Geometry: final body of the model. Coordinates: model frame, mm. Face numbers are marked on the shaded views. A direction names the side the tool comes from. Give positions to 0.01 mm unless a question says otherwise; leave off trailing zeros. Loops run counter-clockwise (first coordinate to the right, second up) from the corner with the lowest first, then second, coordinate; pieces in that order, holes last. Notation, with made-up numbers: (-13, -4) -> (7, -4) arc R14 cw to (7, 23) -> close; hole circle Ø6 at (-21.5, -34). An arc over 180 degrees is marked (long way). One line per question, with ' | ' between items. Start each with the question number.
Item 1: Pin query (flat end, axial travel): P1, Ø10, axis at x = -14, z = 4.5, coming from the +Y side; P2, Ø23, axis at y = 32, z = 0, coming from the -X side; P3, Ø8, axis at x = -27, z = 9, coming from the -Y side. Return the tip coordinate at first contact, or that it passes through.
Item 2: Set-up query: the marked faces 1, 2 and 3. Return all of +Z, -Z, +X, -X, +Y, -Y with unobstructed straight access to the full face (end or side cutting, diameter ignored); none if empty.
Item 3: Section B-B on z = 2. Return loops of the section in (x, y), then the cut area to 3 significant figures.
Item 4: Mould query, pull axis X, two halves, no side actions, for the marked faces 4, 5, 6 and 7. Classes: released by +X, released by -X, zero draft, split by the parting line, or undercut.
Item 5: Material intervals for line 1 along X through (y, z) = (5, -1); line 2 along X through (y, z) = (-1.5, -2); line 3 along Z through (x, y) = (-25, 2.75), sorted ascending. Write a range as [from, to].
Item 6: Section C-C on y = 36. Return loops of the section in (x, z), then the cut area to 3 significant figures.
Item 7: Section A-A on x = -25. Return loops of the section in (y, z).
Item 8: Section D-D on x = -43. Return loops of the section in (y, z).
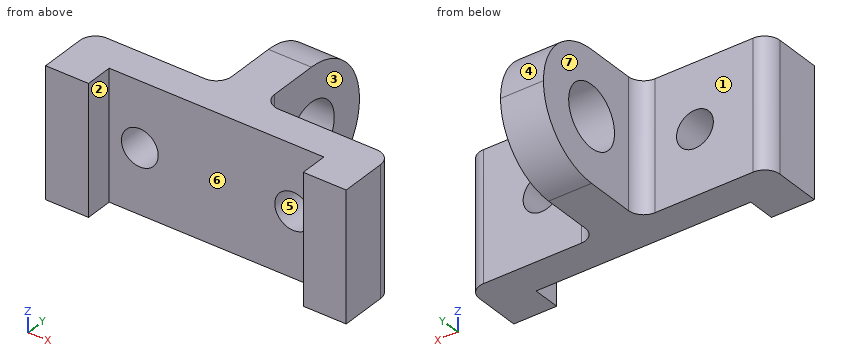
from build123d import *

# Parameters (mm, degrees)
SKETCH2_W               = 98
SKETCH2_H               = 42
BOSS_EXTRUDE1_DEPTH     = 11
SKETCH3_W               = 14
SKETCH3_H               = 42
BOSS_EXTRUDE2_DEPTH     = 9
FILLET1_R               = 5
CUT_EXTRUDE1_DEPTH      = 55.433445601
CUT_EXTRUDE1_DEPTH_BACK = 55.433445601
SKETCH4_R               = 6
SKETCH5_W               = 14
SKETCH5_H               = 42
BOSS_EXTRUDE4_DEPTH     = 53
FILLET2_R               = 21
FILLET3_R               = 5
CUT_EXTRUDE2_DEPTH      = 76.173133499
CUT_EXTRUDE2_DEPTH_BACK = 76.173133499
SKETCH6_R               = 10


with BuildPart() as part:
    # Sketch2 → Boss-Extrude1 (new body)
    with BuildSketch(Plane(origin=(0, 0, 0), x_dir=(1, 0, 0), z_dir=(0, 1, 0))):
        Rectangle(SKETCH2_W, SKETCH2_H)
    extrude(amount=BOSS_EXTRUDE1_DEPTH)

    # Sketch3 → Boss-Extrude2 (add)
    with BuildSketch(Plane(origin=(0, 0, 0), x_dir=(1, 0, 0), z_dir=(0, 1, 0))):
        with Locations((42, 0)):
            Rectangle(SKETCH3_W, SKETCH3_H)
        with Locations((-42, 0)):
            Rectangle(SKETCH3_W, SKETCH3_H)
    extrude(amount=-BOSS_EXTRUDE2_DEPTH)

    # Fillet1
    fillet1_edges = [part.edges().sort_by_distance(p)[0] for p in [
        (-49, 11, 0),
        (49, 11, 0),
    ]]
    fillet(fillet1_edges, radius=FILLET1_R)

    # Sketch4 → Cut-Extrude1 (cut, two sides: drawn at the far end of the back side and taken through both)
    with BuildSketch(Plane(origin=(0, 0, 0), x_dir=(1, 0, 0), z_dir=(0, 1, 0)).offset(-CUT_EXTRUDE1_DEPTH_BACK)):
        with Locations(Location((-25, 0, 0), (0, 0, 270))):
            Circle(SKETCH4_R)
        with Locations(Location((25, 0, 0), (0, 0, 270))):
            Circle(SKETCH4_R)
    extrude(amount=CUT_EXTRUDE1_DEPTH + CUT_EXTRUDE1_DEPTH_BACK, mode=Mode.SUBTRACT)

    # Sketch5 → Boss-Extrude4 (add)
    with BuildSketch(Plane(origin=(0, 0, 0), x_dir=(1, 0, 0), z_dir=(0, 1, 0))):
        Rectangle(SKETCH5_W, SKETCH5_H)
    extrude(amount=BOSS_EXTRUDE4_DEPTH)

    # Fillet2
    fillet2_edges = [part.edges().sort_by_distance(p)[0] for p in [
        (0, 53, -21),
        (0, 53, 21),
    ]]
    fillet(fillet2_edges, radius=FILLET2_R - 0.0001)  # a hair under: the kernel refuses the full size

    # Fillet3
    fillet3_edges = [part.edges().sort_by_distance(p)[0] for p in [
        (7, 11, 0),
        (-7, 11, 0),
    ]]
    fillet(fillet3_edges, radius=FILLET3_R)

    # Sketch6 → Cut-Extrude2 (cut, two sides: drawn at the far end of the back side and taken through both)
    with BuildSketch(Plane(origin=(0, 0, 0), x_dir=(0, 0, -1), z_dir=(1, 0, 0)).offset(-CUT_EXTRUDE2_DEPTH_BACK)):
        with Locations(Location((0, 32, 0), (0, 0, 180))):
            Circle(SKETCH6_R)
    extrude(amount=CUT_EXTRUDE2_DEPTH + CUT_EXTRUDE2_DEPTH_BACK, mode=Mode.SUBTRACT)


solid = part.part
Result sheet:
1) P1: stops at y = 12 | P2: stops at x = -7 | P3: stops at y = 0
2) face 1: +Z, -Z, -X, +Y | face 2: +Z, -Z, -Y | face 3: +Z, -Z, +X, +Y
3) outline: (-49, -9) -> (-35, -9) -> (-35, 0) -> (-30.66, 0) -> (-30.66, 11) -> (-44, 11) arc R5 ccw to (-49, 6) -> close; (-19.34, 0) -> (19.34, 0) -> (19.34, 11) -> (12, 11) arc R5 cw to (7, 16) -> (7, 22.2) -> (-7, 22.2) -> (-7, 16) arc R5 cw to (-12, 11) -> (-19.34, 11) -> close; (-7, 41.8) -> (7, 41.8) -> (7, 52.9) -> (-7, 52.9) -> close; (30.66, 0) -> (35, 0) -> (35, -9) -> (49, -9) -> (49, 6) arc R5 ccw to (44, 11) -> (30.66, 11) -> close | area: 1,390 mm²
4) face 4: zero draft | face 5: undercut | face 6: undercut | face 7: released by -X
5) line 1: x = [-49, -30.92], [-19.08, 19.08], [30.92, 49] | line 2: x = [-49, -35], [35, 49] | line 3: z = [-21, -6], [6, 21]
6) outline: (-7, -20.62) -> (7, -20.62) -> (7, -9.17) -> (-7, -9.17) -> close; (-7, 9.17) -> (7, 9.17) -> (7, 20.62) -> (-7, 20.62) -> close | area: 321 mm²
7) outline: (0, -21) -> (11, -21) -> (11, -6) -> (0, -6) -> close; (0, 6) -> (11, 6) -> (11, 21) -> (0, 21) -> close
8) outline: (-9, -21) -> (11, -21) -> (11, 21) -> (-9, 21) -> close
